Build history of the part. All positions in model axes, mm. Face numbers are marked on the shaded views. Round coordinates to 2 decimals unless told otherwise and drop trailing zeros. Write each loop counter-clockwise with the first axis right and the second up, starting at its lowest first coordinate (ties: lowest second). Pieces come first, ordered by that corner, then holes.
Autodesk Inventor part; units mm, degrees
ref_plane "2CYL_XY" through (1.6, 0, 0) normal (1, 0, 0) x (0, 0, -1)
ref_plane "2CYL_YZ" through (1.6, 0, 0) normal (0, 0, -1) x (0, 1, 0)
ref_plane "2CYL_ZX" through (1.6, 0, 0) normal (0, 1, 0) x (1, 0, 0)
sketch "Sketch_1" plane through (0, 0, 0) normal (0, 1, 0) x (-1, 0, 0)
  line L0 (-3.2, 0) -> (0, 0)
  line L1 (0, 0) -> (0, -6)
  line L2 (0, -6) -> (-3.2, -6)
  line L3 (-3.2, -6) -> (-3.2, 0)
  line L4 (-3.2, 0) -> (0, 0)
revolve "Revolution1" add sketch "Sketch_1" angle 360 about axis through (3.2, 0, 0) along (1, 0, 0)
sketch "Sketch_3" plane through (0, 0, 0) normal (0, 0, 1) x (1, 0, 0)
  line L0 (3.2, 0) -> (0, 0)
  line L1 (-4.45, 10) -> (-4.45, 4.45)
  line L2 (-4.45, 4.45) -> (0, 4.45)
  line L3 (0, 4.45) -> (0.4153, 6)
  line L4 (0.4153, 6) -> (2.7847, 6)
  line L5 (2.7847, 6) -> (3.2, 4.45)
  line L6 (3.2, 4.45) -> (7.65, 4.45)
  line L7 (7.65, 4.45) -> (7.65, 10)
  line L8 (7.65, 10) -> (-4.45, 10)
revolve "Revolution2" cut sketch "Sketch_3" angle 360 about axis through (3.2, 0, 0) along (1, 0, 0)
sketch "Skizze_3" plane through (0, 0, 0) normal (0, 0, 1) x (1, 0, 0)
  line L0 (3.2, 0) -> (0, 0)
  line L1 (0, 0) -> (0, 3)
  line L2 (0, 3) -> (0.5415, 2.4585)
  line L3 (0.5415, 2.4585) -> (2.6585, 2.4585)
  line L4 (2.6585, 2.4585) -> (3.2, 3)
  line L5 (3.2, 3) -> (3.2, 0)
  line L6 (3.2, 0) -> (0, 0)
revolve "Revolution3" cut sketch "Skizze_3" angle 360 about axis through (3.2, 0, 0) along (1, 0, 0)
thread "Thread1"
sketch "Sketch_2" plane through (0, 0, 0) normal (1, 0, 0) x (0, 1, 0)
  line L0 (20, 20) -> (-20, 20)
  line L1 (-20, 20) -> (-20, -20)
  line L2 (-20, -20) -> (20, -20)
  line L3 (20, -20) -> (20, 20)
  line L4 (2.8868, 5) -> (-2.8868, 5)
  line L5 (-2.8868, 5) -> (-5.7735, 0)
  line L6 (-5.7735, 0) -> (-2.8868, -5)
  line L7 (-2.8868, -5) -> (2.8868, -5)
  line L8 (2.8868, -5) -> (5.7735, 0)
  line L9 (5.7735, 0) -> (2.8868, 5)
extrude "Extrusion1" cut sketch "Sketch_2" along normal mid plane 8.4
ref_plane "2CYL_XY" through (1.6, 0, 0) normal (1, 0, 0) x (0, 0, -1)
ref_plane "2CYL_YZ" through (1.6, 0, 0) normal (0, 0, -1) x (0, 1, 0)
ref_plane "2CYL_ZX" through (1.6, 0, 0) normal (0, 1, 0) x (1, 0, 0)
ref_plane "IP1_XY" through (0, 0, 0) normal (1, 0, 0) x (0, 0, -1)
ref_plane "IP1_YZ" through (0, 0, 0) normal (0, 0, -1) x (0, 1, 0)
ref_plane "IP1_ZX" through (0, 0, 0) normal (0, 1, 0) x (1, 0, 0)
ref_plane "IP2_XY" through (3.2, 0, 0) normal (1, 0, 0) x (0, 0, -1)
ref_plane "IP2_YZ" through (3.2, 0, 0) normal (0, 0, -1) x (0, 1, 0)
ref_plane "IP2_ZX" through (3.2, 0, 0) normal (0, 1, 0) x (1, 0, 0)
properties part number "ISO 4035 M6(F)"
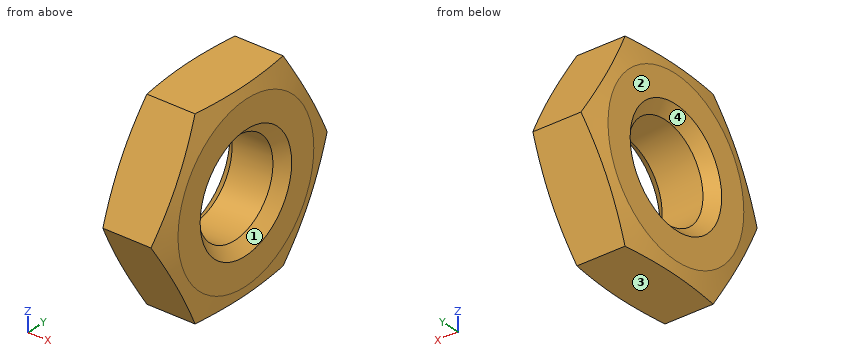
1) Pin check, flat tip, straight feed: pin 1 Ø4 at (y, z) = (0, 0) entering from +X. Stop position of the tip, or through.
Results:
pin 1: passes through
2) Slice it at B-B (x = 1.55). Write the cut outline in (y, z), plus the area to 3 significant figures.
Results:
outline: (-5.77, 0) - (-2.89, -5) - (2.89, -5) - (5.77, 0) - (2.89, 5) - (-2.89, 5) - close; hole circle Ø4.92 at (0, 0)
area: 67.6 mm2
3) Wall check: L1, parallel to Z at x = 1.2, y = 0; L2, parallel to Z at x = 1.4, y = -0.5; L3, parallel to Y at x = 2.6, z = 1.25. Give the ranges that are in metal, low to high.
Results:
L1: z = -5 to -2.46, 2.46 to 5
L2: z = -5 to -2.41, 2.41 to 5
L3: y = -5.05 to -2.12, 2.12 to 5.05
4) Mould opens along Z. For the marked faces 1, 2, 3 and 4 say: released by +Z, released by -Z, zero draft, split by the parting line, or undercut.
Results:
face 1: undercut
face 2: zero draft
face 3: released by -Z
face 4: undercut
5) Slice it at A-A (y = 0). Write the cut outline in (x, z).
Results:
outline: (0, -4.45) - (0.15, -5) - (3.05, -5) - (3.2, -4.45) - (3.2, -3) - (2.66, -2.46) - (0.54, -2.46) - (0, -3) - close; (0, 3) - (0.54, 2.46) - (2.66, 2.46) - (3.2, 3) - (3.2, 4.45) - (3.05, 5) - (0.15, 5) - (0, 4.45) - close
